Build history of the part. All positions in model axes, mm. A direction names the side the tool comes from. Give positions to 0.01 mm unless a question says otherwise; leave off trailing zeros. Order: outer loops, then holes, each group sorted by start corner. A loop starts at its lowest first (then second) coordinate and runs counter-clockwise, first axis right, second up. Notation, with made-up numbers: (56.5, 59) - (92.5, 59) arc R7 cw to (92.5, 70) - close; hole circle Ø2 at (3, 64.25). An arc over 180 degrees is marked (long way). One line per item, written item: value.
```python
from build123d import *

# Parameters (mm, degrees)
CROQUIS1_W              = 66
CROQUIS1_H              = 50
CROQUIS1_W_2            = 30
CROQUIS1_H_2            = 43
SALIENTE_EXTRUIR1_DEPTH = 15
CROQUIS2_R              = 1.5
CROQUIS2_W              = 10
CROQUIS2_H              = 12
CORTAR_EXTRUIR1_DEPTH   = 67
CROQUIS3_W              = 2
CROQUIS3_H              = 12
CORTAR_EXTRUIR2_DEPTH   = 12


with BuildPart() as part:
    # Croquis1 → Saliente-Extruir1 (new body)
    with BuildSketch(Plane.XY):
        with Locations((33, 25)):
            Rectangle(CROQUIS1_W, CROQUIS1_H)
        with Locations((33, 23.5)):
            Rectangle(CROQUIS1_W_2, CROQUIS1_H_2, mode=Mode.SUBTRACT)
    extrude(amount=SALIENTE_EXTRUIR1_DEPTH)

    # Croquis2 → Cortar-Extruir1 (cut, through all)
    with BuildSketch(Plane.ZY):
        with Locations((7.5, 42)):
            Circle(CROQUIS2_R)
        with Locations((7.5, 8)):
            Circle(CROQUIS2_R)
        with Locations((10, 25)):
            Rectangle(CROQUIS2_W, CROQUIS2_H)
    extrude(amount=-CORTAR_EXTRUIR1_DEPTH, mode=Mode.SUBTRACT)

    # Croquis3 → Cortar-Extruir2 (cut)
    with BuildSketch(Plane.XY.offset(15)):
        with Locations((5, 44)):
            Rectangle(CROQUIS3_W, CROQUIS3_H)
        with Locations((61, 44)):
            Rectangle(CROQUIS3_W, CROQUIS3_H)
        with Locations((5, 6)):
            Rectangle(CROQUIS3_W, CROQUIS3_H)
        with Locations((61, 6)):
            Rectangle(CROQUIS3_W, CROQUIS3_H)
    extrude(amount=-CORTAR_EXTRUIR2_DEPTH, mode=Mode.SUBTRACT)


solid = part.part
```
(1) Slice it at A-A, the plane x = 55.5. Give the cut face in (y, z), and give its area (3 significant figures).
Completed:
outline: (0, 0) - (50, 0) - (50, 15) - (31, 15) - (31, 5) - (19, 5) - (19, 15) - (0, 15) - close; hole circle Ø3 at (8, 7.5); hole circle Ø3 at (42, 7.5)
area: 616 mm²
(2) Pull direction X, two halves, no side cores. Call faces 4 (the face through (66, 25, 4)), 5 (the face through (18, 23, 4)), 6 (the face through (63.972, 40.536, 7.175)): +X half, -X half, draft (parallel to the pull), parting line (faces both ways), or undercut.
Completed:
face 4: +X half
face 5: undercut
face 6: draft
(3) Slice it at C-C, the plane y = 8. Count the separate pieces of the cut face and the enclosed holes in it, and give its area (3 significant figures).
Completed:
separate pieces: 6
enclosed holes: 0
area: 396 mm²
(4) 3-axis set-ups, long thin cutter, end or side, ignore diameter. For faces 1 (the face through (9, 31, 10)), 2 (the face through (33, 45, 7)), 3 (the face through (6, 6, 9)): which of +Z, -Z, +X, -X, +Y, -Y reach the whole face in a straight line?
Completed:
face 1: +Z, +X, -X
face 2: +Z, -Z
face 3: +Z, -Y
(5) Slice it at D-D, the plane x = 35. Give the cut face in (y, z).
Completed:
outline: (0, 0) - (2, 0) - (2, 15) - (0, 15) - close; (45, 0) - (50, 0) - (50, 15) - (45, 15) - close
(6) Drill centre lines: line 1 (X direction, y = 10.5, z = 6.5); line 2 (Y direction, x = 56.75, z = 7.5); line 3 (Y direction, x = 31, z = 14). Where is each one in solid material? Low to high.
Completed:
line 1: 0 to 4, 6 to 18, 48 to 60, 62 to 66
line 2: 0 to 6.5, 9.5 to 19, 31 to 40.5, 43.5 to 50
line 3: 0 to 2, 45 to 50
(7) Pin check, flat tips, straight feed: P1, Ø4, axis at y = 8, z = 7.5, coming from the +X side; P2, Ø1.6, axis at x = 61, z = 8, coming from the -Y side; P3, Ø1, axis at x = 61, z = 9.5, coming from the +Y side; P4, Ø0.6, axis at x = 61, y = 45.5, coming from the +Z side. Stop position of each tip, or through.
Completed:
P1: x = 66
P2: y = 12
P3: y = 38
P4: z = 3
